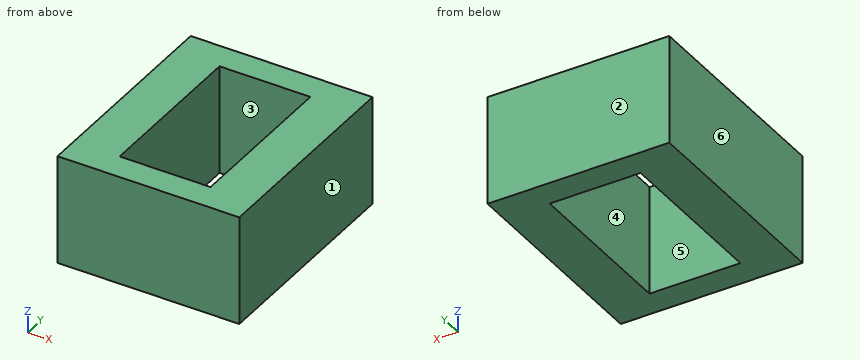
```python
from build123d import *

# Parameters (mm, degrees)
F0_W     = 5
F0_H     = 6
F0_W_2   = 2.5
F0_H_2   = 4.5
F1_DEPTH = 3


with BuildPart() as f1:
    # F0 (on Top) → F1 (new body)
    with BuildSketch(Plane.XY):
        Rectangle(F0_W, F0_H)
        Rectangle(F0_W_2, F0_H_2, mode=Mode.SUBTRACT)
    extrude(amount=F1_DEPTH)


solid = f1.part
```
Can you work these out from the model? Positions are in its coordinate system, mm. Face numbers are marked on the shaded views. A direction names the side the tool comes from. Coordinates: 2 decimals unless noted, no trailing zeros. Write each loop counter-clockwise with the first axis right and the second up, starting at its lowest first coordinate (ties: lowest second). Pieces come first, ordered by that corner, then holes. Notation, with made-up numbers: (28.5, 18) - (68.5, 18) arc R31 cw to (68.5, 50) - close; hole circle Ø4 at (-32.5, -1.5). An arc over 180 degrees is marked (long way). Return JSON: item names as keys, results as strings.
Q1. On a 3-axis mill with a long thin cutter (end or side, diameter ignored), from which of +Z, -Z, +X, -X, +Y, -Y can I reach the whole of each face in a straight line? I mean the marked faces 5 and 6. Say none if no direction works.
Computed values:
{"face 5": "+Z, -Z", "face 6": "+Z, -Z, -X, +Y, -Y"}
Q2. If we section it at A-A (x = -0.3): Please give me the cut outline in (y, z).
Computed values:
{"outline": "(-3, 0) - (-2.25, 0) - (-2.25, 3) - (-3, 3) - close; (2.25, 0) - (3, 0) - (3, 3) - (2.25, 3) - close"}
Q3. If we section it at B-B (y = 0.8): Please give me the cut outline in (x, z).
Computed values:
{"outline": "(-2.5, 0) - (-1.25, 0) - (-1.25, 3) - (-2.5, 3) - close; (1.25, 0) - (2.5, 0) - (2.5, 3) - (1.25, 3) - close"}
Q4. Please list where these lines run through material, in increasing order: L1, parallel to Y at x = -0.1, z = 1.8; L2, parallel to X at y = -0.15, z = 2.4. Write a range as from..to.
Computed values:
{"L1": "y = -3..-2.25, 2.25..3", "L2": "x = -2.5..-1.25, 1.25..2.5"}
Q5. Thinking about a two-plate mould opening in X: for the marked faces 1, 2, 3 and 4, which applies, +X half, -X half, draft (parallel to the pull), parting line (faces both ways), or undercut?
Computed values:
{"face 1": "+X half", "face 2": "draft", "face 3": "undercut", "face 4": "undercut"}
Q6. If we section it at C-C (z = 2.65): Please give me the cut outline in (x, y).
Computed values:
{"outline": "(-2.5, -3) - (2.5, -3) - (2.5, 3) - (-2.5, 3) - close; hole (-1.25, -2.25) - (1.25, -2.25) - (1.25, 2.25) - (-1.25, 2.25) - close"}
